Input: part model. Units: mm. Frame: model coordinates. Give positions to 0.01 mm unless a question says otherwise; leave off trailing zeros. Answer in a Markdown table with one row per item. Add a question column.
1. Ray query, line 1 (Y direction, x = 50, z = 7.25) (3 decimals); line 2 (Y direction, x = -40, z = 6) (3 decimals); line 3 (Y direction, x = 21, z = 9.75). Return the intervals inside material, ascending. Write a range as [from, to].
2. Contact query for a flat-ended pin moving along its axis: pin 1 (3 mm diameter, centred on x = 60, y = 10, fed in from -Z). Output: stop coordinate, or through.
3. Section query A-A on z = 8.25. Count the separate pieces of the cut face and the enclosed holes in it, and give its area (3 significant figures).
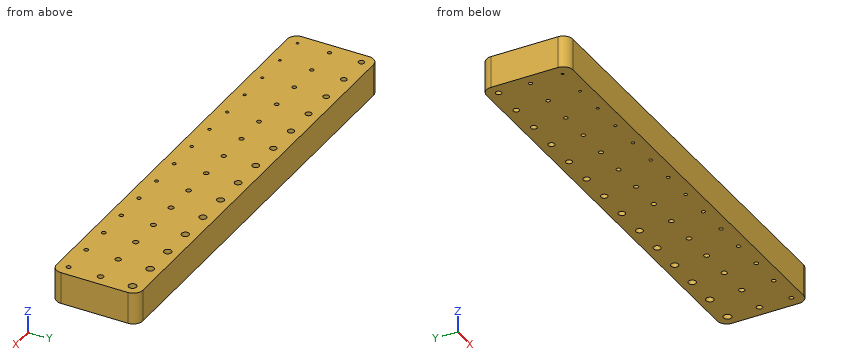
Autodesk Fusion 360 part; units mm, degrees
sketch "Sketch1" plane through (0, 0, 0) normal (0, 0, 1) x (1, 0, 0)
  circle A0 centre (0, 0) radius 0.74
  circle A1 centre (10, 0) radius 0.765
  circle A2 centre (20, 0) radius 0.79
  circle A3 centre (30, 0) radius 0.815
  circle A4 centre (40, 0) radius 0.84
  line L0 (0, 0) -> (10, 0) construction
  line L1 (10, 0) -> (20, 0) construction
  line L2 (20, 0) -> (30, 0) construction
  line L3 (30, 0) -> (40, 0) construction
  circle A5 centre (50, 0) radius 0.865
  circle A6 centre (60, 0) radius 0.89
  circle A7 centre (70, 0) radius 0.915
  line L4 (40, 0) -> (50, 0) construction
  line L5 (50, 0) -> (60, 0) construction
  line L6 (60, 0) -> (70, 0) construction
  line L7 (-50, 0) -> (-40, 0) construction
  line L8 (-40, 0) -> (-30, 0) construction
  circle A8 centre (-40, 0) radius 0.64
  line L9 (-10, 0) -> (0, 0) construction
  circle A9 centre (-50, 0) radius 0.615
  circle A10 centre (-30, 0) radius 0.665
  circle A11 centre (-60, 0) radius 0.59
  circle A12 centre (-20, 0) radius 0.69
  line L10 (-30, 0) -> (-20, 0) construction
  line L11 (-60, 0) -> (-50, 0) construction
  line L12 (-20, 0) -> (-10, 0) construction
  circle A13 centre (-10, 0) radius 0.715
  line L13 (0, 0) -> (0, 10) construction
  circle A14 centre (-40, 10) radius 0.95
  line L14 (-50, 10) -> (-40, 10) construction
  line L15 (20, 10) -> (30, 10) construction
  circle A15 centre (20, 10) radius 1.1
  line L16 (-30, 10) -> (-20, 10) construction
  circle A16 centre (0, 10) radius 1.05
  circle A17 centre (-50, 10) radius 0.925
  line L17 (-60, 10) -> (-50, 10) construction
  line L18 (40, 10) -> (50, 10) construction
  line L19 (-40, 10) -> (-30, 10) construction
  circle A18 centre (10, 10) radius 1.075
  circle A19 centre (-30, 10) radius 0.975
  line L20 (-20, 10) -> (-10, 10) construction
  circle A20 centre (60, 10) radius 1.2
  circle A21 centre (70, 10) radius 1.225
  line L21 (60, 10) -> (70, 10) construction
  circle A22 centre (30, 10) radius 1.125
  line L22 (50, 10) -> (60, 10) construction
  circle A23 centre (40, 10) radius 1.15
  circle A24 centre (50, 10) radius 1.175
  line L23 (30, 10) -> (40, 10) construction
  circle A25 centre (-10, 10) radius 1.025
  line L24 (-10, 10) -> (0, 10) construction
  line L25 (0, 10) -> (10, 10) construction
  circle A26 centre (-20, 10) radius 1
  circle A27 centre (-60, 10) radius 0.9
  line L26 (10, 10) -> (20, 10) construction
  line L27 (0, 0) -> (0, -10) construction
  line L28 (0, -10) -> (10, -10) construction
  circle A28 centre (30, -10) radius 0.6
  circle A29 centre (20, -10) radius 0.575
  circle A30 centre (40, -10) radius 0.625
  line L29 (50, -10) -> (60, -10) construction
  circle A31 centre (70, -10) radius 0.7
  circle A32 centre (10, -10) radius 0.55
  line L30 (20, -10) -> (30, -10) construction
  circle A33 centre (0, -10) radius 0.525
  line L31 (-20, -10) -> (-10, -10) construction
  circle A34 centre (-10, -10) radius 0.5
  circle A35 centre (-20, -10) radius 0.475
  line L32 (-10, -10) -> (0, -10) construction
  circle A36 centre (-40, -10) radius 0.425
  circle A37 centre (-60, -10) radius 0.375
  line L33 (-60, -10) -> (-50, -10) construction
  line L34 (-30, -10) -> (-20, -10) construction
  circle A38 centre (-50, -10) radius 0.4
  line L35 (-40, -10) -> (-30, -10) construction
  line L36 (-50, -10) -> (-40, -10) construction
  circle A39 centre (-30, -10) radius 0.45
  circle A40 centre (50, -10) radius 0.65
  line L37 (10, -10) -> (20, -10) construction
  line L38 (40, -10) -> (50, -10) construction
  line L39 (60, -10) -> (70, -10) construction
  line L40 (30, -10) -> (40, -10) construction
  circle A41 centre (60, -10) radius 0.675
  line L41 (73.5, 13.5) -> (-63.5, 13.5)
  line L42 (-63.5, 13.5) -> (-63.5, -13.5)
  line L43 (-63.5, -13.5) -> (73.5, -13.5)
  line L44 (73.5, -13.5) -> (73.5, 13.5)
  line L45 (73.5, 13.5) -> (-63.5, -13.5) construction
  line L46 (-63.5, 13.5) -> (73.5, -13.5) construction
  point P0 (-60, 0)
  point P1 (-60, 10)
  point P2 (0, 10)
  point P3 (0, 10)
  point P4 (0, -10)
  point P5 (-60, -10)
  point P6 (0, -10)
  point P7 (0, -10)
  point P8 (5, 0)
  dimension "d1" = 1.48
  dimension "d2" = 10
  dimension "d3" = 1.53
  dimension "d4" = 1.58
  dimension "d5" = 1.63
  dimension "d6" = 1.68
  dimension "d7" = 1.73
  dimension "d8" = 1.78
  dimension "d9" = 1.83
  dimension "d10" = 1.18
  dimension "d11" = 10
  dimension "d12" = 1.23
  dimension "d13" = 1.28
  dimension "d14" = 1.33
  dimension "d15" = 1.38
  dimension "d16" = 1.43
  dimension "d18" = 10
  dimension "d19" = 2.1
  dimension "d20" = 10
  dimension "d21" = 2.15
  dimension "d22" = 2.2
  dimension "d23" = 2.25
  dimension "d24" = 2.3
  dimension "d25" = 2.35
  dimension "d26" = 2.4
  dimension "d27" = 2.45
  dimension "d28" = 1.8
  dimension "d29" = 10
  dimension "d30" = 1.85
  dimension "d31" = 1.9
  dimension "d32" = 1.95
  dimension "d33" = 2
  dimension "d34" = 2.05
  dimension "d35" = 1.05
  dimension "d36" = 10
  dimension "d37" = 1.1
  dimension "d38" = 1.15
  dimension "d39" = 1.2
  dimension "d40" = 1.25
  dimension "d41" = 1.3
  dimension "d42" = 1.35
  dimension "d43" = 1.4
  dimension "d44" = 0.75
  dimension "d45" = 10
  dimension "d46" = 0.8
  dimension "d47" = 0.85
  dimension "d48" = 0.9
  dimension "d49" = 0.95
  dimension "d50" = 1
  dimension "d51" = 137
  dimension "d52" = 27
extrude "Extrude1" add sketch "Sketch1" along normal blind 10
fillet "Fillet1" radius 3 4 edges at (73.5, -13.5, 5) (73.5, 13.5, 5) (-63.5, -13.5, 5) (-63.5, 13.5, 5)
equation "d2 = d18"
equation "d3 = d1 + 0.05 mm"
equation "d4 = d3 + 0.05 mm"
equation "d5 = d4 + 0.05 mm"
equation "d6 = d5 + 0.05 mm"
equation "d7 = d6 + 0.05 mm"
equation "d8 = d7 + 0.05 mm"
equation "d9 = d8 + 0.05 mm"
equation "d10 = d12 - 0.05 mm"
equation "d11 = d2"
equation "d12 = d13 - 0.05 mm"
equation "d13 = d14 - 0.05 mm"
equation "d14 = d15 - 0.05 mm"
equation "d15 = d16 - 0.05 mm"
equation "d16 = d1 - 0.05 mm"
equation "d20 = d2"
equation "d21 = d19 + 0.05 mm"
equation "d22 = d19 + 0.1 mm"
equation "d23 = d19 + 0.15 mm"
equation "d24 = d19 + 0.2 mm"
equation "d25 = d19 + 0.25 mm"
equation "d26 = d19 + 0.3 mm"
equation "d27 = d19 + 0.35 mm"
equation "d28 = d19 - 0.3 mm"
equation "d29 = d2"
equation "d30 = d19 - 0.25 mm"
equation "d31 = d19 - 0.2 mm"
equation "d32 = d19 - 0.15 mm"
equation "d33 = d19 - 0.1 mm"
equation "d34 = d19 - 0.05 mm"
equation "d36 = d2"
equation "d37 = d35 + 0.05 mm"
equation "d38 = d37 + 0.05 mm"
equation "d39 = d38 + 0.05 mm"
equation "d40 = d39 + 0.05 mm"
equation "d41 = d40 + 0.05 mm"
equation "d42 = d41 + 0.05 mm"
equation "d43 = d42 + 0.05 mm"
equation "d44 = d46 - 0.05 mm"
equation "d45 = d2"
equation "d46 = d47 - 0.05 mm"
equation "d47 = d48 - 0.05 mm"
equation "d48 = d49 - 0.05 mm"
equation "d49 = d50 - 0.05 mm"
equation "d50 = d35 - 0.05 mm"
Answer:
| question | item | result |
|---|---|---|
| 1 | line 1 | y = [-13.5, -10.65], [-9.35, -0.865], [0.865, 8.825], [11.175, 13.5] |
| 1 | line 2 | y = [-13.5, -10.425], [-9.575, -0.64], [0.64, 9.05], [10.95, 13.5] |
| 1 | line 3 | y = [-13.5, 9.54], [10.46, 13.5] |
| 2 | pin 1 | stops at z = 0 |
| 3 | separate pieces | 1 |
| 3 | enclosed holes | 42 |
| 3 | area | 3,600 mm² |
